```python
from build123d import *

# Parameters (mm, degrees)
F1_DEPTH = 30
F3_DEPTH = 10
F5_DEPTH = 10
F6_SIZE  = 1.2


with BuildPart() as f1:
    # F0 (on Top) → F1 (new body)
    with BuildSketch(Plane.XY):
        with BuildLine():
            Line((-9.216308, -17.411032), (30.691593, -14.698203))
            ThreePointArc((30.691593, -14.698203), (36.514619, 6.635995), (24.655298, 25.301797))
            Line((24.655298, 25.301797), (5.084314, 21.18153))
            ThreePointArc((5.084314, 21.18153), (1.133073, 17.897067), (-3.807032, 19.309641))
            Line((-3.807032, 19.309641), (-13.592523, 17.249507))
            ThreePointArc((-13.592523, 17.249507), (-17.660185, -0.870611), (-9.216308, -17.411032))
        make_face()
        with BuildLine():
            ThreePointArc((-8.23102, -14.738054), (-15.082961, -0.526675), (-11.955391, 14.937177))
            Line((-11.955391, 14.937177), (-4.457272, 16.515751))
            ThreePointArc((-4.457272, 16.515751), (1.668708, 15.35284), (6.805824, 18.886964))
            Line((6.805824, 18.886964), (24.089435, 22.525672))
            ThreePointArc((24.089435, 22.525672), (33.940977, 6.266214), (29.353638, -12.183153))
            Line((29.353638, -12.183153), (-8.23102, -14.738054))
        make_face(mode=Mode.SUBTRACT)
    extrude(amount=F1_DEPTH)

    # F2 (on face) → F3 (cut)
    with BuildSketch(Plane(origin=(0, 0, 0), x_dir=(1, 0, 0), z_dir=(0, 0, -1))):
        with BuildLine():
            Line((30.691593, 14.698203), (-9.216308, 17.411032))
            ThreePointArc((-9.216308, 17.411032), (-17.660185, 0.870611), (-13.592523, -17.249507))
            Line((-13.592523, -17.249507), (-3.807032, -19.309641))
            ThreePointArc((-3.807032, -19.309641), (1.133073, -17.897067), (5.084314, -21.18153))
            Line((5.084314, -21.18153), (24.655298, -25.301797))
            ThreePointArc((24.655298, -25.301797), (36.514619, -6.635995), (30.691593, 14.698203))
        make_face()
        with BuildLine():
            ThreePointArc((6.045536, -19.953206), (1.421492, -16.527099), (-4.191416, -17.798027))
            Line((-4.191416, -17.798027), (-12.719125, -16.002694))
            ThreePointArc((-12.719125, -16.002694), (-16.272457, 0.685365), (-8.694441, 15.972326))
            Line((-8.694441, 15.972326), (29.979829, 13.343356))
            ThreePointArc((29.979829, 13.343356), (35.128806, -6.436932), (24.358737, -23.808673))
            Line((24.358737, -23.808673), (6.045536, -19.953206))
        make_face(mode=Mode.SUBTRACT)
    extrude(amount=-F3_DEPTH, mode=Mode.SUBTRACT)

    # F4 (on face) → F5 (cut)
    with BuildSketch(Plane.XY.offset(30)):
        with BuildLine():
            Line((-3.807032, 19.309641), (-13.592523, 17.249507))
            ThreePointArc((-13.592523, 17.249507), (-17.660185, -0.870611), (-9.216308, -17.411032))
            Line((-9.216308, -17.411032), (30.691593, -14.698203))
            ThreePointArc((30.691593, -14.698203), (36.514619, 6.635995), (24.655298, 25.301797))
            Line((24.655298, 25.301797), (5.084314, 21.18153))
            ThreePointArc((5.084314, 21.18153), (1.133073, 17.897067), (-3.807032, 19.309641))
        make_face()
        with BuildLine():
            ThreePointArc((-8.694441, -15.972326), (-16.272457, -0.685365), (-12.719125, 16.002694))
            Line((-12.719125, 16.002694), (-4.191416, 17.798027))
            ThreePointArc((-4.191416, 17.798027), (1.421492, 16.527099), (6.045536, 19.953206))
            Line((6.045536, 19.953206), (24.358737, 23.808673))
            ThreePointArc((24.358737, 23.808673), (35.128806, 6.436932), (29.979829, -13.343356))
            Line((29.979829, -13.343356), (-8.694441, -15.972326))
        make_face(mode=Mode.SUBTRACT)
    extrude(amount=-F5_DEPTH, mode=Mode.SUBTRACT)

    # F6
    f6_edges = [f1.edges().sort_by_distance(p)[0] for p in [
        (-16.272457, -0.685365, 20),
        (-8.455271, 16.90036, 20),
        (1.421492, 16.527099, 20),
        (15.202137, 21.88094, 20),
        (35.128806, 6.436932, 20),
        (10.642694, -14.657841, 20),
        (15.202137, 21.88094, 10),
        (35.128806, 6.436932, 10),
        (1.421492, 16.527099, 10),
        (-8.455271, 16.90036, 10),
        (-16.272457, -0.685365, 10),
        (10.642694, -14.657841, 10),
    ]]
    chamfer(f6_edges, length=F6_SIZE)


solid = f1.part
```
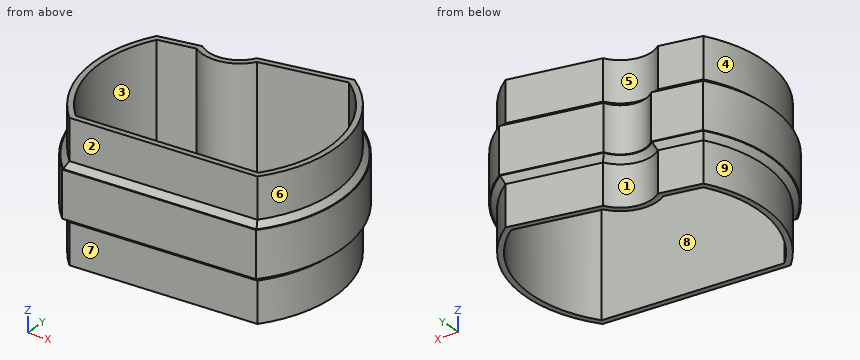
The model under review builds one solid part; all positions refer to its coordinate system, in mm. Face numbers are marked on the shaded views. A direction names the side the tool comes from. Coordinates: 2 decimals unless noted, no trailing zeros. Loops run counter-clockwise (first coordinate to the right, second up) from the corner with the lowest first, then second, coordinate; pieces in that order, holes last. Notation, with made-up numbers: (-1.75, -6) -> (34.25, -6) arc R35 ccw to (34.25, 27) -> close; hole circle Ø10 at (-32.75, 87.25). An arc over 180 degrees is marked (long way). Answer as CSV lines item,"result".
Item 1: Take a section at B-B, the plane x = -6.5. State the section outline as (y, z) points, and give its area (3 significant figures).
Results below:
outline,"(-17.23, 10) -> (-17.03, 10) -> (-15.82, 8.8) -> (-15.82, 0) -> (-14.62, 0) -> (-14.62, 30) -> (-15.82, 30) -> (-15.82, 21.2) -> (-17.03, 20) -> (-17.23, 20) -> close; (16.09, 0) -> (17.31, 0) -> (17.31, 8.8) -> (18.54, 10) -> (18.74, 10) -> (18.74, 20) -> (18.54, 20) -> (17.31, 21.2) -> (17.31, 30) -> (16.09, 30) -> close"
area,"104 mm2"
Item 2: Insertion check: pin 1 (2 mm diameter, centred on y = 16, z = 21.5, fed in from +X); pin 2 (3 mm diameter, centred on x = 2, z = 10.5, fed in from -Y); pin 3 (10 mm diameter, centred on y = 15.5, z = 10.5, fed in from +X). Each pin has a flat end and moves straight along its axis. Give the tip position at first contact, or say it passes through.
Results below:
pin 1,"stops at x = 32.62"
pin 2,"stops at y = -16.75"
pin 3,"stops at x = 35.64"
Item 3: Machinability: for the marked faces 5, 6, 7, 8 and 9, which of the approach directions +Z, -Z, +X, -X, +Y, -Y give a long, thin tool a straight path to every point of the face, cutting with its end or side? Answer none if there is none.
Results below:
face 5,"+Z, +Y"
face 6,"+Z, +X"
face 7,"-Z, +X, -Y"
face 8,"+Z, -Z"
face 9,"-Z, -X"
Item 4: For L1, parallel to X at y = 7, z = 7.25; L2, parallel to X at y = -8, z = 4; L3, parallel to Y at x = 23, z = 22, list the stretches that pass through material, from the lowest coordinate up.
Results below:
L1,"x = -16.09 to -14.87, 33.82 to 35.04"
L2,"x = -14.23 to -12.91, 31.86 to 33.18"
L3,"y = -13.82 to -12.62, 22.3 to 23.52"
Item 5: Take a section at A-A, the plane z = 14. State the section outline as (x, y) points.
Results below:
outline,"(-13.59, 17.25) arc R27.35 ccw to (-9.22, -17.41) -> (30.69, -14.7) arc R27.35 ccw to (24.66, 25.3) -> (5.08, 21.18) arc R5.5 cw to (-3.81, 19.31) -> close; hole (-11.96, 14.94) arc R24.75 ccw to (-8.23, -14.74) -> (29.35, -12.18) arc R24.75 ccw to (24.09, 22.53) -> (6.81, 18.89) arc R8.1 cw to (-4.46, 16.52) -> close"
Item 6: Draft analysis for pull direction Y (two halves, no side actions). For the marked faces 1, 2, 3 and 4, state which applies: +Y half, -Y half, draft (parallel to the pull), parting line (faces both ways), or undercut.
Results below:
face 1,"+Y half"
face 2,"-Y half"
face 3,"undercut"
face 4,"parting line"
